```python
from build123d import *

# Parameters (mm, degrees)
BOSS_EXTRUDE1_DEPTH = 34.925
SKETCH2_R           = 2.54
CUT_EXTRUDE1_DEPTH  = 99.014466407
SKETCH4_W           = 50.8
SKETCH4_H           = 28.575
CUT_EXTRUDE3_DEPTH  = 99.014466407
FILLET1_R           = 5.08
SKETCH5_R           = 6.35
CUT_EXTRUDE4_DEPTH  = 22.225


with BuildPart() as part:
    # Sketch1 → Boss-Extrude1 (new body)
    with BuildSketch(Plane.XY):
        Polygon((0, 0), (0, 50.8), (25.4, 50.8), (25.4, 25.4), (76.2, 25.4), (76.2, 0), align=None)
    extrude(amount=BOSS_EXTRUDE1_DEPTH)

    # Sketch2 → Cut-Extrude1 (cut, through all)
    with BuildSketch(Plane.XY.offset(34.925)):
        with Locations((12.7, 38.1)):
            Circle(SKETCH2_R)
        with Locations((12.7, 12.7)):
            Circle(SKETCH2_R)
        with Locations((38.1, 12.7)):
            Circle(SKETCH2_R)
        with Locations((63.5, 12.7)):
            Circle(SKETCH2_R)
    extrude(amount=-CUT_EXTRUDE1_DEPTH, mode=Mode.SUBTRACT)

    # Sketch4 → Cut-Extrude3 (cut, through all)
    with BuildSketch(Plane.XZ):
        with Locations((50.8, 20.6375)):
            Rectangle(SKETCH4_W, SKETCH4_H)
    extrude(amount=-CUT_EXTRUDE3_DEPTH, mode=Mode.SUBTRACT)

    # Fillet1
    fillet1_edges = [part.edges().sort_by_distance(p)[0] for p in [
        (25.4, 25.4, 3.175),
        (25.4, 12.7, 6.35),
    ]]
    fillet(fillet1_edges, radius=FILLET1_R)

    # Sketch5 → Cut-Extrude4 (cut)
    with BuildSketch(Plane(origin=(0, 0, 0), x_dir=(-1, 0, 0), z_dir=(0, 0, -1))):
        with Locations((-12.7, 38.1)):
            Circle(SKETCH5_R)
    extrude(amount=-CUT_EXTRUDE4_DEPTH, mode=Mode.SUBTRACT)


solid = part.part
```
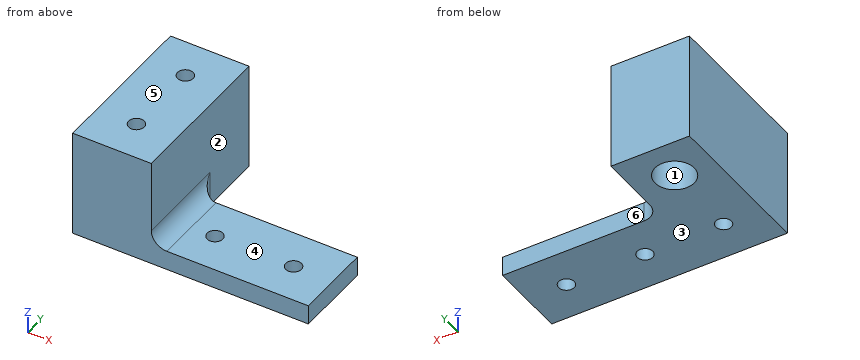
Work out the finished part from the listing and answer in its coordinate system (mm). Face numbers are marked on the shaded views. A direction names the side the tool comes from. Coordinates: 2 decimals unless noted, no trailing zeros. Write each loop counter-clockwise with the first axis right and the second up, starting at its lowest first coordinate (ties: lowest second). Pieces come first, ordered by that corner, then holes. Notation, with made-up numbers: (49.5, -25) - (54.5, -25) arc R9 ccw to (54.5, -9) - close; hole circle Ø3 at (-37, 14). An arc over 180 degrees is marked (long way). Answer as a JSON object with one key per item and string values.
Q1. Find section C-C (y = 12.7). Write down the section's boundary in (x, z) (3 decimals), plus the area to 3 significant figures.
Results list:
{"outline": "(0, 0) - (10.16, 0) - (10.16, 34.925) - (0, 34.925) - close; (15.24, 0) - (35.56, 0) - (35.56, 6.35) - (30.48, 6.35) arc R5.08 cw to (25.4, 11.43) - (25.4, 34.925) - (15.24, 34.925) - close; (40.64, 0) - (60.96, 0) - (60.96, 6.35) - (40.64, 6.35) - close; (66.04, 0) - (76.2, 0) - (76.2, 6.35) - (66.04, 6.35) - close", "area": "973 mm^2"}
Q2. Find section D-D (z = 24). Write down the section's boundary in (x, y).
Results list:
{"outline": "(0, 0) - (25.4, 0) - (25.4, 50.8) - (0, 50.8) - close; hole circle Ø5.08 at (12.7, 12.7); hole circle Ø5.08 at (12.7, 38.1)"}
Q3. Given pin 1 Ø4.5 at (x, y) = (38.1, 12.7) entering from +Z; pin 2 Ø3 at (x, z) = (64, 3) entering from +Y; pin 3 Ø6.5 at (x, y) = (63.5, 12.7) entering from +Z; pin 4 Ø3 at (y, z) = (33.5, 20) entering from +X, each flat-ended and moving along its own axis, determine where each tip first touches the part or whether it passes through.
Results list:
{"pin 1": "passes through", "pin 2": "stops at y = 25.4", "pin 3": "stops at z = 6.35", "pin 4": "stops at x = 25.4"}
Q4. For a pull along X with two mould halves and no side action, classify the marked faces 1, 2 and 3 as pulls with the +X half, pulls with the -X half, needs draft (parallel to the pull), parting line crosses it, or undercut.
Results list:
{"face 1": "undercut", "face 2": "pulls with the +X half", "face 3": "needs draft"}
Q5. Consider L1, parallel to Y at x = 12, z = 9; L2, parallel to X at y = 12, z = 3; L3, parallel to Y at x = 38, z = 3. Determine where each line is inside the solid, lowest interval first. Write a range as from..to.
Results list:
{"L1": "y = 0..10.26, 15.14..31.79, 44.41..50.8", "L2": "x = 0..10.26, 15.14..35.66, 40.54..61.06, 65.94..76.2", "L3": "y = 0..10.16, 15.24..25.4"}
Q6. Find section A-A (y = 38.1). Write down the section's boundary in (x, z) (3 decimals).
Results list:
{"outline": "(0, 0) - (6.35, 0) - (6.35, 22.225) - (10.16, 22.225) - (10.16, 34.925) - (0, 34.925) - close; (15.24, 22.225) - (19.05, 22.225) - (19.05, 0) - (25.4, 0) - (25.4, 34.925) - (15.24, 34.925) - close"}
Q7. Find section B-B (x = 63.5). Write down the section's boundary in (y, z), plus the area to 3 significant figures.
Results list:
{"outline": "(0, 0) - (10.16, 0) - (10.16, 6.35) - (0, 6.35) - close; (15.24, 0) - (25.4, 0) - (25.4, 6.35) - (15.24, 6.35) - close", "area": "129 mm^2"}
Q8. Which of the six approach directions +Z, -Z, +X, -X, +Y, -Y give full straight-line access (tool end or side, diameter ignored) to the marked faces 4, 5 and 6?
Results list:
{"face 4": "+Z, +X, +Y, -Y", "face 5": "+Z, +X, -X, +Y, -Y", "face 6": "+Z, -Z, +X, +Y"}
